CAD build for the part. Positions are in the model's coordinates, mm. Round coordinates to 2 decimals unless told otherwise and drop trailing zeros. Order: outer loops, then holes, each group sorted by start corner. A loop starts at its lowest first (then second) coordinate and runs counter-clockwise, first axis right, second up. Notation, with made-up numbers: M 77.25,42.5 L 124.25,42.5 A35 cw 124.25,76.5 Z; hole C 22.25,31 d4. An arc over 180 degrees is marked long. Answer as a JSON object with one key per item and string values.
```python
from build123d import *

# Parameters (mm, degrees)
MB1_2_R        = 6.049999109
MB1_2_R_2      = 6.050000891
EXTRUDE1_DEPTH = 100


with BuildPart() as part:
    # MB1-2 → Extrude1 (new body)
    with BuildSketch(Plane.XY):
        Polygon((-13, -33.265685), (-11.634315, -33.265685), (-7.5, -29.131371165), (-7.5, -20.868628835), (-11.634315, -16.734315), (-13, -16.734315), (-13, -21), (-15, -21), (-15, -4), (-13, -4), (-13, -8.265685), (-11.634315, -8.265685), (-7.5, -4.131371165), (-7.5, 4.131371165), (-11.634315, 8.265685), (-13, 8.265685), (-13, 4), (-15, 4), (-15, 21), (-13, 21), (-13, 16.734315), (-11.634315, 16.734315), (-7.5, 20.868628835), (-7.5, 29.131371165), (-11.634315, 33.265685), (-13, 33.265685), (-13, 29), (-15, 29), (-15, 50), (-4, 50), (-4, 48), (-8.265685, 48), (-8.265685, 46.634315), (-4.131371165, 42.5), (4.131371165, 42.5), (8.265685, 46.634315), (8.265685, 48), (4, 48), (4, 50), (15, 50), (15, 29), (13, 29), (13, 33.265685), (11.634315, 33.265685), (7.5, 29.131371165), (7.5, 20.868628835), (11.634315, 16.734315), (13, 16.734315), (13, 21), (15, 21), (15, 4), (13, 4), (13, 8.265685), (11.634315, 8.265685), (7.5, 4.131371165), (7.5, -4.131371165), (11.634315, -8.265685), (13, -8.265685), (13, -4), (15, -4), (15, -21), (13, -21), (13, -16.734315), (11.634315, -16.734315), (7.5, -20.868628835), (7.5, -29.131371165), (11.634315, -33.265685), (13, -33.265685), (13, -29), (15, -29), (15, -50), (4, -50), (4, -48), (8.265685, -48), (8.265685, -46.634315), (4.131371165, -42.5), (-4.131371165, -42.5), (-8.265685, -46.634315), (-8.265685, -48), (-4, -48), (-4, -50), (-15, -50), (-15, -29), (-13, -29), align=None)
        with Locations((0, -24.999996952)):
            Circle(MB1_2_R, mode=Mode.SUBTRACT)
        with Locations((0, 24.999996952)):
            Circle(MB1_2_R_2, mode=Mode.SUBTRACT)
        with BuildLine():
            Line((5.74819726, -30.346094347), (6.169137939, -30.346093939))
            Line((6.169137939, -30.346093939), (11.123044, -35.3))
            Line((11.123044, -35.3), (13.2, -35.3))
            Line((13.2, -35.3), (13.2, -48.5))
            Line((13.2, -48.5), (10.3, -48.5))
            Line((10.3, -48.5), (10.3, -46.123043785))
            Line((10.3, -46.123043785), (4.876954686, -40.7))
            Line((4.876954686, -40.7), (-4.876954686, -40.7))
            Line((-4.876954686, -40.7), (-10.3, -46.123043785))
            Line((-10.3, -46.123043785), (-10.3, -48.5))
            Line((-10.3, -48.5), (-13.2, -48.5))
            Line((-13.2, -48.5), (-13.2, -35.3))
            Line((-13.2, -35.3), (-11.123044, -35.3))
            Line((-11.123044, -35.3), (-6.169138347, -30.346094347))
            Line((-6.169138347, -30.346094347), (-5.74819688, -30.346094756))
            ThreePointArc((-5.74819688, -30.346094756), (2.79e-07, -32.849998806), (5.74819726, -30.346094347))
        make_face(mode=Mode.SUBTRACT)
        with BuildLine():
            Line((6.169138347, 30.346094347), (5.74819688, 30.346094756))
            ThreePointArc((5.74819688, 30.346094756), (-2.79e-07, 32.849998806), (-5.74819726, 30.346094347))
            Line((-5.74819726, 30.346094347), (-6.169137939, 30.346093939))
            Line((-6.169137939, 30.346093939), (-11.123044, 35.3))
            Line((-11.123044, 35.3), (-13.2, 35.3))
            Line((-13.2, 35.3), (-13.2, 48.5))
            Line((-13.2, 48.5), (-10.3, 48.5))
            Line((-10.3, 48.5), (-10.3, 46.123043785))
            Line((-10.3, 46.123043785), (-4.876954686, 40.7))
            Line((-4.876954686, 40.7), (4.876954686, 40.7))
            Line((4.876954686, 40.7), (10.3, 46.123043785))
            Line((10.3, 46.123043785), (10.3, 48.5))
            Line((10.3, 48.5), (13.2, 48.5))
            Line((13.2, 48.5), (13.2, 35.3))
            Line((13.2, 35.3), (11.123044, 35.3))
            Line((11.123044, 35.3), (6.169138347, 30.346094347))
        make_face(mode=Mode.SUBTRACT)
        with BuildLine():
            Line((-11.123044, -14.7), (-5.947034494, -19.876009506))
            ThreePointArc((-5.947034494, -19.876009506), (0, -17.149999078), (5.947034494, -19.876009506))
            Line((5.947034494, -19.876009506), (11.123044, -14.7))
            Line((11.123044, -14.7), (13.5, -14.7))
            Line((13.5, -14.7), (13.5, -10.3))
            Line((13.5, -10.3), (11.123044, -10.3))
            Line((11.123044, -10.3), (5.947034535, -5.123990535))
            ThreePointArc((5.947034535, -5.123990535), (5.181974313, -5.896578485), (4.3175, -6.556043))
            ThreePointArc((4.3175, -6.556043), (3.079734534, -6.258736768), (3.375725, -5.020656))
            ThreePointArc((3.375725, -5.020656), (6.050002522, 0), (3.375725, 5.020656))
            ThreePointArc((3.375725, 5.020656), (3.078919, 6.259237), (4.3175, 6.556043))
            ThreePointArc((4.3175, 6.556043), (5.181974313, 5.896578485), (5.947034535, 5.123990535))
            Line((5.947034535, 5.123990535), (11.123044, 10.3))
            Line((11.123044, 10.3), (13.5, 10.3))
            Line((13.5, 10.3), (13.5, 14.7))
            Line((13.5, 14.7), (11.123044, 14.7))
            Line((11.123044, 14.7), (5.947034494, 19.876009506))
            ThreePointArc((5.947034494, 19.876009506), (0, 17.149999078), (-5.947034494, 19.876009506))
            Line((-5.947034494, 19.876009506), (-11.123044, 14.7))
            Line((-11.123044, 14.7), (-13.5, 14.7))
            Line((-13.5, 14.7), (-13.5, 10.3))
            Line((-13.5, 10.3), (-11.123044, 10.3))
            Line((-11.123044, 10.3), (-5.947034535, 5.123990535))
            ThreePointArc((-5.947034535, 5.123990535), (-5.181974313, 5.896578485), (-4.3175, 6.556043))
            ThreePointArc((-4.3175, 6.556043), (-3.079734534, 6.258736768), (-3.375725, 5.020656))
            ThreePointArc((-3.375725, 5.020656), (-6.049998461, 0), (-3.375725, -5.020656))
            ThreePointArc((-3.375725, -5.020656), (-3.079734534, -6.258736768), (-4.3175, -6.556043))
            ThreePointArc((-4.3175, -6.556043), (-5.181974313, -5.896578485), (-5.947034535, -5.123990535))
            Line((-5.947034535, -5.123990535), (-11.123044, -10.3))
            Line((-11.123044, -10.3), (-13.5, -10.3))
            Line((-13.5, -10.3), (-13.5, -14.7))
            Line((-13.5, -14.7), (-11.123044, -14.7))
        make_face(mode=Mode.SUBTRACT)
    extrude(amount=-EXTRUDE1_DEPTH)


solid = part.part
```
Item 1: Two-plate mould, pull along X, no slides. Class faces 1 (the flat face through (0, 42.5, -49)), 2 (the flat face through (-15, 12, -49)), 3 (the flat face through (10, -50, -49)), 4 (the flat face through (15, 13, -49)): released by +X, released by -X, zero draft, split by the parting line, or undercut.
Worked answers:
{"face 1": "undercut", "face 2": "released by -X", "face 3": "zero draft", "face 4": "released by +X"}
Item 2: Saw through at B-B on z = -39.5. State how many separate pieces and enclosed holes the cut face has, and give its area (3 significant figures).
Worked answers:
{"separate pieces": "1", "enclosed holes": "5", "area": "845 mm2"}
Item 3: Wall check: line 1 along Y through (x, z) = (13.75, -75.5); line 2 along X through (y, z) = (0.5, -61); line 3 along X through (y, z) = (43, -81). Give the ranges that are in metal, low to high. Write a range as [from, to].
Worked answers:
{"line 1": "y = [-50, -29], [-21, -4], [4, 21], [29, 50]", "line 2": "x = [-7.5, -6.03], [6.03, 7.5]", "line 3": "x = [-15, -13.2], [-7.18, -4.63], [4.63, 7.18], [13.2, 15]"}
Item 4: Saw through at A-A on x = 0. List the corners of the cut face in (y, z).
Worked answers:
{"outline": "M -42.5,-100 L -40.7,-100 L -40.7,0 L -42.5,0 Z; M -32.85,-100 L -31.05,-100 L -31.05,0 L -32.85,0 Z; M -18.95,-100 L -17.15,-100 L -17.15,0 L -18.95,0 Z; M 17.15,-100 L 18.95,-100 L 18.95,0 L 17.15,0 Z; M 31.05,-100 L 32.85,-100 L 32.85,0 L 31.05,0 Z; M 40.7,-100 L 42.5,-100 L 42.5,0 L 40.7,0 Z"}
Item 5: Drop flat-ended pins along their axis: pin 1 Ø3 at (x, y) = (3, 26) entering from +Z; pin 2 Ø3 at (x, z) = (-1, -20.5) entering from +Y. Give the stop position or say it passes through.
Worked answers:
{"pin 1": "passes through", "pin 2": "stops at y = 42.5"}
